from build123d import *

# Parameters (mm, degrees)
F0_R            = 47.5
F1_DEPTH        = 8.7
F2_R            = 34
F3_DEPTH        = 15.4
F5_DEPTH        = 15.401
F6_R            = 20
F7_DEPTH        = 15.401
F9_D            = 9
F9_COPIES_COUNT = 6


# Not quite as in the source:
# - a pattern or mirror of a feature is missing from the dataset's text; its kind, count and spacing are read off the source's solid


with BuildPart() as f1:
    # F0 (on Top) → F1 (new body)
    with BuildSketch(Plane.XY):
        Circle(F0_R)
    extrude(amount=-F1_DEPTH)

    # F2 (on face) → F3 (join)
    with BuildSketch(Plane.XY):
        Circle(F2_R)
    extrude(amount=-F3_DEPTH)

    # F4 (on face) → F5 (cut, through all)
    with BuildSketch(Plane.XY):
        with BuildLine():
            Line((-21.2132034356, 42.5), (21.2132034356, 42.5))
            ThreePointArc((21.2132034356, 42.5), (0, 47.5), (-21.2132034356, 42.5))
        make_face()
    extrude(amount=-F5_DEPTH, mode=Mode.SUBTRACT)

    # F6 (on face) → F7 (cut, through all)
    with BuildSketch(Plane.XY):
        Circle(F6_R)
    extrude(amount=-F7_DEPTH, mode=Mode.SUBTRACT)

    # F9 (through all)
    with Locations(Plane.XY):
        with Locations((-40, 0)):
            f9 = Hole(F9_D / 2)

    # F9_copies: F9 ×6 about axis
    f9_copies_axis = Axis((0, 0, 0), (0, 0, 1))
    for i in range(1, F9_COPIES_COUNT):
        add(f9.rotate(f9_copies_axis, i * 360 / F9_COPIES_COUNT), mode=Mode.SUBTRACT)


solid = f1.part
Check sheet for the modelled part. Datum: model origin and axes. Units: mm. A direction names the side the tool comes from. Round coordinates to 2 decimals unless told otherwise and drop trailing zeros. Loops run counter-clockwise (first coordinate to the right, second up) from the corner with the lowest first, then second, coordinate; pieces in that order, holes last. Notation, with made-up numbers: (37.25, 58.25) - (67.25, 58.25) arc R17 ccw to (67.25, 84.25) - close; hole circle Ø8 at (78.5, -39.5). An arc over 180 degrees is marked (long way). Answer as CSV lines item,"result". Start each with the question number.
Item 1: Section check D-D (y = -9). Record the boundary of the cut face in (x, z).
Item 2: Set-up check for faces 1 (the cylindrical face through (18.28, 28.67, -12)), 2 (the flat face through (0, 42.5, -4)): record each of +Z, -Z, +X, -X, +Y, -Y from which the full face is reachable in a straight line by a thin tool's end or side.
Item 3: Section check A-A (x = 0). Record the boundary of the cut face in (y, z), and give its area (3 significant figures).
Item 4: Depth check by flat-ended pin: P1, Ø3, axis at y = 29.5, z = -7.5, coming from the +X side; P2, Ø1, axis at x = 22.5, y = -1, coming from the +Z side; P3, Ø10.5, axis at x = -20, y = 34.64, coming from the -Z side; P4, Ø6, axis at y = 23.5, z = -4, coming from the +X side. Enter the tip coordinate at first touch or a pass-through.
Item 5: Release check for a two-part mould opening along Y. For faces 3 (the cylindrical face through (-1.781, -47.467, -4.289)), 4 (the cylindrical face through (17.581, -30.847, -4.411)), 5 (the flat face through (15, -15, -15.4)), 6 (the cylindrical face through (44.292, -1.352, -4.411)) record: +Y half, -Y half, draft (parallel to the pull), parting line (faces both ways), or undercut.
Item 6: Scan lines: line 1 (X direction, y = -38, z = -2); line 2 (X direction, y = 32, z = -8.5); line 3 (Y direction, x = 22, z = -3.75). Record each from-to range of solid material in increasing order. Write a range as [from, to].
Item 7: Section check C-C (x = -18.5). Record the boundary of the cut face in (y, z), and give its area (3 significant figures).
Item 8: Section check B-B (y = 0). Record the boundary of the cut face in (x, z).
Report:
1,outline,"(-46.64, -8.7) - (-32.79, -8.7) - (-32.79, -15.4) - (-17.86, -15.4) - (-17.86, 0) - (-46.64, 0) - close; (17.86, -15.4) - (32.79, -15.4) - (32.79, -8.7) - (46.64, -8.7) - (46.64, 0) - (17.86, 0) - close"
2,face 1,"-Z"
2,face 2,"+Z, -Z, +X, -X, +Y"
3,outline,"(-47.5, -8.7) - (-34, -8.7) - (-34, -15.4) - (-20, -15.4) - (-20, 0) - (-47.5, 0) - close; (20, -15.4) - (34, -15.4) - (34, -8.7) - (42.5, -8.7) - (42.5, 0) - (20, 0) - close"
3,area,"623 mm2"
4,P1,"stops at x = 38.37"
4,P2,"stops at z = 0"
4,P3,"stops at z = -8.7"
4,P4,"stops at x = 42.85"
5,face 3,"parting line"
5,face 4,"undercut"
5,face 5,"draft"
5,face 6,"undercut"
6,line 1,"x = [-28.5, -22.99], [-17.01, 17.01], [22.99, 28.5]"
6,line 2,"x = [-35.1, -23.64], [-16.36, 16.36], [23.64, 35.1]"
6,line 3,"y = [-42.1, -38.67], [-30.61, 30.61], [38.67, 42.1]"
7,outline,"(-43.75, -8.7) - (-38.88, -8.7) - (-38.88, 0) - (-43.75, 0) - close; (-30.4, -8.7) - (-28.53, -8.7) - (-28.53, -15.4) - (-7.6, -15.4) - (-7.6, 0) - (-30.4, 0) - close; (7.6, -15.4) - (28.53, -15.4) - (28.53, -8.7) - (30.4, -8.7) - (30.4, 0) - (7.6, 0) - close; (38.88, -8.7) - (42.5, -8.7) - (42.5, 0) - (38.88, 0) - close"
7,area,"751 mm2"
8,outline,"(-47.5, -8.7) - (-44.5, -8.7) - (-44.5, 0) - (-47.5, 0) - close; (-35.5, -8.7) - (-34, -8.7) - (-34, -15.4) - (-20, -15.4) - (-20, 0) - (-35.5, 0) - close; (20, -15.4) - (34, -15.4) - (34, -8.7) - (35.5, -8.7) - (35.5, 0) - (20, 0) - close; (44.5, -8.7) - (47.5, -8.7) - (47.5, 0) - (44.5, 0) - close"
